Input: part model. Units: mm. Frame: model coordinates. Face numbers are marked on the shaded views. A direction names the side the tool comes from. Give positions to 0.01 mm unless a question says otherwise; leave off trailing zeros. Order: outer loops, then holes, each group sorted by start corner. A loop starts at its lowest first (then second) coordinate and runs counter-clockwise, first axis right, second up. Notation, with made-up numbers: (-9.5, 59) - (20.5, 59) arc R20 cw to (20.5, 78) - close; hole circle Ø3 at (2, 11.5). An arc over 180 degrees is marked (long way). Answer in a Markdown table with one row per item. Add a question column.
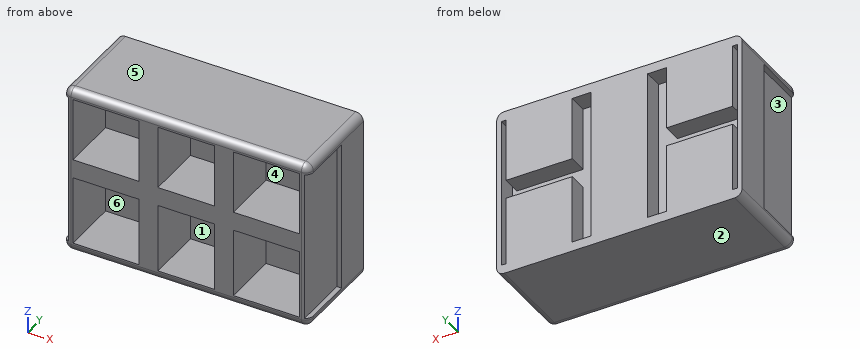
from build123d import *

# Parameters (mm, degrees)
F0_W     = 3.175
F0_H     = 6.35
F0_W_2   = 6.35
F0_W_3   = 44.45
F0_W_4   = 15.0601655953
F0_W_5   = 5.811475683
F0_W_6   = 6.888524317
F0_W_7   = 10.3398344047
F0_H_2   = 42.6130002154
F0_H_3   = 46.2869997846
F1_DEPTH = 50.8
F0_H_4   = 52.6369997846
F0_H_5   = 48.9630002154
F2_DEPTH = 12.7
F3_F1_R  = 5.08
F3_F2_R  = 5.08
F3_F3_R  = 5.08
F3_F4_R  = 5.08


with BuildPart() as f1:
    # F0 (on Front) → F1 (new body)
    with BuildSketch(Plane.XZ):
        Polygon((0, -58.9869997846), (0, -52.6369997846), (-5.811475683, -52.6369997846), (-20.8716412783, -52.6369997846), (-27.2216412783, -52.6369997846), (-33.5716412783, -52.6369997846), (-78.0216412783, -52.6369997846), (-78.0216412783, -58.9869997846), align=None)
        with Locations((-79.6091412783, 52.1380002154)):
            Rectangle(F0_W, F0_H)
        with Locations((-82.7841412783, 52.1380002154)):
            Rectangle(F0_W, F0_H)
        Polygon((-5.811475683, 48.9630002154), (0, 48.9630002154), (0, 55.3130002154), (-78.0216412783, 55.3130002154), (-78.0216412783, 48.9630002154), (-33.5716412783, 48.9630002154), (-27.2216412783, 48.9630002154), (-20.8716412783, 48.9630002154), align=None)
        Polygon((0, 55.3130002154), (0, 48.9630002154), (6.888524317, 48.9630002154), (17.2283587217, 48.9630002154), (23.5783587217, 48.9630002154), (29.9283587217, 48.9630002154), (74.3783587217, 48.9630002154), (74.3783587217, 55.3130002154), align=None)
        Polygon((80.7283587217, 55.3130002154), (77.5533587217, 55.3130002154), (77.5533587217, 48.9315246976), (80.7283587217, 48.9000491798), align=None)
        Polygon((77.5533587217, 55.3130002154), (74.3783587217, 55.3130002154), (74.3783587217, 48.9630002154), (77.5533587217, 48.9315246976), align=None)
        Polygon((6.888524317, -52.6369997846), (0, -52.6369997846), (0, -58.9869997846), (80.7283587217, -58.9869997846), (80.7283587217, -52.6369997846), (77.5533587217, -52.6369997846), (74.3783587217, -52.6369997846), (29.9283587217, -52.6369997846), (23.5783587217, -52.6369997846), (17.2283587217, -52.6369997846), align=None)
        with Locations((-82.7841412783, -55.8119997846)):
            Rectangle(F0_W, F0_H)
        with Locations((-79.6091412783, -55.8119997846)):
            Rectangle(F0_W, F0_H)
        with Locations((-30.3966412783, 3.175)):
            Rectangle(F0_W_2, F0_H)
        with Locations((-24.0466412783, 3.175)):
            Rectangle(F0_W_2, F0_H)
        with Locations((-30.3966412783, -3.175)):
            Rectangle(F0_W_2, F0_H)
        with Locations((-24.0466412783, -3.175)):
            Rectangle(F0_W_2, F0_H)
        with Locations((20.4033587217, -3.175)):
            Rectangle(F0_W_2, F0_H)
        with Locations((20.4033587217, 3.175)):
            Rectangle(F0_W_2, F0_H)
        with Locations((26.7533587217, 3.175)):
            Rectangle(F0_W_2, F0_H)
        with Locations((26.7533587217, -3.175)):
            Rectangle(F0_W_2, F0_H)
        with Locations((-55.7966412783, 3.175)):
            Rectangle(F0_W_3, F0_H)
        with Locations((-55.7966412783, -3.175)):
            Rectangle(F0_W_3, F0_H)
        with Locations((-13.3415584806, 3.175)):
            Rectangle(F0_W_4, F0_H)
        with Locations((-13.3415584806, -3.175)):
            Rectangle(F0_W_4, F0_H)
        with Locations((-2.9057378415, 3.175)):
            Rectangle(F0_W_5, F0_H)
        with Locations((-2.9057378415, -3.175)):
            Rectangle(F0_W_5, F0_H)
        with Locations((3.4442621585, -3.175)):
            Rectangle(F0_W_6, F0_H)
        with Locations((3.4442621585, 3.175)):
            Rectangle(F0_W_6, F0_H)
        with Locations((12.0584415194, -3.175)):
            Rectangle(F0_W_7, F0_H)
        with Locations((12.0584415194, 3.175)):
            Rectangle(F0_W_7, F0_H)
        with Locations((52.1533587217, 3.175)):
            Rectangle(F0_W_3, F0_H)
        with Locations((52.1533587217, -3.175)):
            Rectangle(F0_W_3, F0_H)
        with Locations((-30.3966412783, 27.6565001077)):
            Rectangle(F0_W_2, F0_H_2)
        with Locations((-24.0466412783, 27.6565001077)):
            Rectangle(F0_W_2, F0_H_2)
        with Locations((-30.3966412783, -29.4934998923)):
            Rectangle(F0_W_2, F0_H_3)
        with Locations((-24.0466412783, -29.4934998923)):
            Rectangle(F0_W_2, F0_H_3)
        with Locations((20.4033587217, 27.6565001077)):
            Rectangle(F0_W_2, F0_H_2)
        with Locations((26.7533587217, 27.6565001077)):
            Rectangle(F0_W_2, F0_H_2)
        with Locations((20.4033587217, -29.4934998923)):
            Rectangle(F0_W_2, F0_H_3)
        with Locations((26.7533587217, -29.4934998923)):
            Rectangle(F0_W_2, F0_H_3)
        Polygon((77.5533587217, 48.9315246976), (74.3783587217, 48.9630002154), (74.3783587217, 6.35), (74.3783587217, 0), (77.5533587217, 0), align=None)
        Polygon((77.5533587217, 0), (74.3783587217, 0), (74.3783587217, -6.35), (74.3783587217, -52.6369997846), (77.5533587217, -52.6369997846), align=None)
        Polygon((-78.0216412783, 6.35), (-78.0216412783, 48.9630002154), (-81.1966412783, 48.9630002154), (-81.1966412783, 0), (-78.0216412783, 0), align=None)
        Polygon((-81.1966412783, -52.6369997846), (-78.0216412783, -52.6369997846), (-78.0216412783, -6.35), (-78.0216412783, 0), (-81.1966412783, 0), align=None)
    extrude(amount=F1_DEPTH)

    # F0 (on Front) → F2 (join, symmetric)
    with BuildSketch(Plane.XZ):
        with Locations((-2.9057378415, 3.175)):
            Rectangle(F0_W_5, F0_H)
        with Locations((3.4442621585, -3.175)):
            Rectangle(F0_W_6, F0_H)
        with Locations((-2.9057378415, -3.175)):
            Rectangle(F0_W_5, F0_H)
        with Locations((3.4442621585, 3.175)):
            Rectangle(F0_W_6, F0_H)
        with Locations((-2.9057378415, 27.6565001077)):
            Rectangle(F0_W_5, F0_H_2)
        with Locations((3.4442621585, 27.6565001077)):
            Rectangle(F0_W_6, F0_H_2)
        with Locations((3.4442621585, -29.4934998923)):
            Rectangle(F0_W_6, F0_H_3)
        with Locations((-2.9057378415, -29.4934998923)):
            Rectangle(F0_W_5, F0_H_3)
        with Locations((-13.3415584806, -3.175)):
            Rectangle(F0_W_4, F0_H)
        with Locations((-13.3415584806, 3.175)):
            Rectangle(F0_W_4, F0_H)
        with Locations((12.0584415194, 3.175)):
            Rectangle(F0_W_7, F0_H)
        with Locations((12.0584415194, -3.175)):
            Rectangle(F0_W_7, F0_H)
        Polygon((0, 55.3130002154), (0, 48.9630002154), (6.888524317, 48.9630002154), (17.2283587217, 48.9630002154), (23.5783587217, 48.9630002154), (29.9283587217, 48.9630002154), (74.3783587217, 48.9630002154), (74.3783587217, 55.3130002154), align=None)
        Polygon((-5.811475683, 48.9630002154), (0, 48.9630002154), (0, 55.3130002154), (-78.0216412783, 55.3130002154), (-78.0216412783, 48.9630002154), (-33.5716412783, 48.9630002154), (-27.2216412783, 48.9630002154), (-20.8716412783, 48.9630002154), align=None)
        with Locations((12.0584415194, 27.6565001077)):
            Rectangle(F0_W_7, F0_H_2)
        with Locations((-13.3415584806, 27.6565001077)):
            Rectangle(F0_W_4, F0_H_2)
        Polygon((0, -58.9869997846), (0, -52.6369997846), (-5.811475683, -52.6369997846), (-20.8716412783, -52.6369997846), (-27.2216412783, -52.6369997846), (-33.5716412783, -52.6369997846), (-78.0216412783, -52.6369997846), (-78.0216412783, -58.9869997846), align=None)
        Polygon((6.888524317, -52.6369997846), (0, -52.6369997846), (0, -58.9869997846), (80.7283587217, -58.9869997846), (80.7283587217, -52.6369997846), (77.5533587217, -52.6369997846), (74.3783587217, -52.6369997846), (29.9283587217, -52.6369997846), (23.5783587217, -52.6369997846), (17.2283587217, -52.6369997846), align=None)
        with Locations((12.0584415194, -29.4934998923)):
            Rectangle(F0_W_7, F0_H_3)
        with Locations((-13.3415584806, -29.4934998923)):
            Rectangle(F0_W_4, F0_H_3)
        with Locations((-79.6091412783, 52.1380002154)):
            Rectangle(F0_W, F0_H)
        Polygon((77.5533587217, 55.3130002154), (74.3783587217, 55.3130002154), (74.3783587217, 48.9630002154), (77.5533587217, 48.9315246976), align=None)
        with Locations((-79.6091412783, -55.8119997846)):
            Rectangle(F0_W, F0_H)
        with Locations((-55.7966412783, 27.6565001077)):
            Rectangle(F0_W_3, F0_H_2)
        with Locations((-82.7841412783, 52.1380002154)):
            Rectangle(F0_W, F0_H)
        with Locations((52.1533587217, 27.6565001077)):
            Rectangle(F0_W_3, F0_H_2)
        Polygon((80.7283587217, 55.3130002154), (77.5533587217, 55.3130002154), (77.5533587217, 48.9315246976), (80.7283587217, 48.9000491798), align=None)
        with Locations((79.1408587217, -26.3184998923)):
            Rectangle(F0_W, F0_H_4)
        with Locations((-55.7966412783, -29.4934998923)):
            Rectangle(F0_W_3, F0_H_3)
        with Locations((-82.7841412783, -55.8119997846)):
            Rectangle(F0_W, F0_H)
        with Locations((52.1533587217, -29.4934998923)):
            Rectangle(F0_W_3, F0_H_3)
        with Locations((-82.7841412783, 24.4815001077)):
            Rectangle(F0_W, F0_H_5)
        Polygon((80.7283587217, 48.9000491798), (77.5533587217, 48.9315246976), (77.5533587217, 0), (80.7283587217, 0), align=None)
        with Locations((-82.7841412783, -26.3184998923)):
            Rectangle(F0_W, F0_H_4)
    extrude(amount=F2_DEPTH, both=True)

    # F3: fillet of radius 5.08 on 10 edges, made by hand

    # F3_f1
    f3_f1_edges = [f1.edges().sort_by_distance(p)[0] for p in [
        (80.7283587217, -19.05, 55.3130002154),
    ]]
    fillet(f3_f1_edges, radius=F3_F1_R)

    # F3_f2
    f3_f2_edges = [f1.edges().sort_by_distance(p)[0] for p in [
        (-84.3716412783, -19.05, 55.3130002154),
    ]]
    fillet(f3_f2_edges, radius=F3_F2_R)

    # F3_f3
    f3_f3_edges = [f1.edges().sort_by_distance(p)[0] for p in [
        (-1.8216412783, -50.8, 55.3130002154),
    ]]
    fillet(f3_f3_edges, radius=F3_F3_R)

    # F3_f4
    f3_f4_edges = [f1.edges().sort_by_distance(p)[0] for p in [
        (-1.8216412783, -50.8, -58.9869997846),
    ]]
    fillet(f3_f4_edges, radius=F3_F4_R)


solid = f1.part
Q1. Access query for the marked faces 5 and 6. Directions: +Z, -Z, +X, -X, +Y, -Y. A direction counts if a zero-diameter tool reaches every point of the face in a straight line with its end or side. Return the directions, or none.
Q2. Pull-direction query (X, two-part tool) for the marked faces 1, 2, 3 and 4; classes: +X half, -X half, draft (parallel to the pull), parting line (faces both ways), or undercut.
Q3. Section B-B, the plane x = 34. Return loops of the section in (y, z).
Q4. Section C-C, the plane x = -26.5. Return loops of the section in (y, z), then the cut area to 3 significant figures.
Q5. Section A-A, the plane y = 7.5. State how many separate pieces and enclosed holes the cut face has, then the cut area to 3 significant figures.
Q6. Contact query for flat-ended pins moving along their axis: P1, Ø19, axis at y = -32.5, z = -38, coming from the +X side; P2, Ø19, axis at y = -32, z = -40, coming from the -X side; P3, Ø1.6, axis at x = -83, y = -33.5, coming from the +Z side; P4, Ø6, axis at y = -13.5, z = 27.5, coming from the -X side. Output: stop coordinate, or through.
Q7. Line query: probe 1 along X at (y, z) = (-23, -14); probe 2 along X at (y, z) = (8.5, 33.5); probe 3 along Z at (x, y) = (-43.5, -20). Output: solid intervals per line, ascending.
Computed:
| question | item | result |
|---|---|---|
| 1 | face 5 | +Z, +X, -X, +Y, -Y |
| 1 | face 6 | -Y |
| 2 | face 1 | undercut |
| 2 | face 2 | draft |
| 2 | face 3 | -X half |
| 2 | face 4 | undercut |
| 3 | outline | (-50.8, -53.91) arc R5.08 ccw to (-45.72, -58.99) - (12.7, -58.99) - (12.7, -6.35) - (0, -6.35) - (0, 6.35) - (12.7, 6.35) - (12.7, 55.31) - (-45.72, 55.31) arc R5.08 ccw to (-50.8, 50.23) - (-50.8, 48.96) - (-12.7, 48.96) - (-12.7, 6.35) - (-50.8, 6.35) - (-50.8, -6.35) - (-12.7, -6.35) - (-12.7, -52.64) - (-50.8, -52.64) - close |
| 4 | outline | (-50.8, -53.91) arc R5.08 ccw to (-45.72, -58.99) - (12.7, -58.99) - (12.7, -52.64) - (0, -52.64) - (0, 48.96) - (12.7, 48.96) - (12.7, 55.31) - (-45.72, 55.31) arc R5.08 ccw to (-50.8, 50.23) - close |
| 4 | area | 5,960 mm^2 |
| 5 | separate pieces | 1 |
| 5 | enclosed holes | 2 |
| 5 | area | 14,500 mm^2 |
| 6 | P1 | stops at x = 77.55 |
| 6 | P2 | stops at x = -81.2 |
| 6 | P3 | stops at z = 54.4 |
| 6 | P4 | stops at x = -84.37 |
| 7 | probe 1 | x = -81.2 to -78.02, -33.57 to -20.87, 17.23 to 29.93, 74.38 to 77.55 |
| 7 | probe 2 | x = -84.37 to -81.2, -78.02 to -33.57, -20.87 to 17.23, 29.93 to 74.38, 77.55 to 80.73 |
| 7 | probe 3 | z = -58.99 to -52.64, -6.35 to 6.35, 48.96 to 55.31 |
